Geometry check sheet. Reference: the model listing, model coordinates, mm. Face numbers are marked on the shaded views. A direction names the side the tool comes from. Round coordinates to 2 decimals unless told otherwise and drop trailing zeros. Order: outer loops, then holes, each group sorted by start corner. A loop starts at its lowest first (then second) coordinate and runs counter-clockwise, first axis right, second up.
(1) Thickness scan on L1, parallel to Z at x = 64, y = 22; L2, parallel to X at y = 3.15, z = 0; L3, parallel to Z at x = -75, y = 1.8. Record the ranges inside material, lowest first.
(2) Draft check along Z on the marked faces 1, 2 and 3. Enter one of: pulls with the +Z half, pulls with the -Z half, needs draft (parallel to the pull), parting line crosses it, or undercut.
(3) Cross-section at B-B on y = 19.25. Enter the section's corners in (x, z).
(4) Cross-section at A-A on z = 0. Enter the section's corners in (x, y).
(5) Set-up check for the marked faces 4 and 5: record each of +Z, -Z, +X, -X, +Y, -Y from which the full face is reachable in a straight line by a thin tool's end or side.
(6) Gauge pin test, flat ends, axial feed: P1, Ø5, axis at x = 62.5, z = 68.5, coming from the +Y side; P2, Ø7.5, axis at y = 20.5, z = 50.5, coming from the -X side; P3, Ø3, axis at y = 3, z = 17.5, coming from the -X side; P4, Ø2, axis at x = -8.5, z = -74.5, coming from the -Y side. Record the tip position at first contact, or that the pin passes through.
from build123d import *

# Parameters (mm, degrees)
BOSS_EXTRUDE2_DEPTH      = 4
CUT_EXTRUDE3_DEPTH       = 157.951186811
CUT_EXTRUDE3_DEPTH_BACK  = 157.951186811
SKETCH3_R                = 1.6
CUT_EXTRUDE6_DEPTH       = 157.951186811
CUT_EXTRUDE6_DEPTH_BACK  = 157.951186811
SKETCH6_R                = 17.5
SKETCH8_R                = 1.5
CUT_EXTRUDE7_DEPTH       = 4
CIRPATTERN1_COUNT        = 4
SKETCH10_R               = 1.55
CUT_EXTRUDE8_DEPTH       = 4
SKETCH11_W               = 146
SKETCH11_H               = 43.5
SKETCH11_W_2             = 140
SKETCH11_H_2             = 38
BOSS_EXTRUDE4_DEPTH      = 25
SKETCH12_W               = 90
SKETCH12_H               = 3
CUT_EXTRUDE9_DEPTH       = 25
FILLET1_R                = 2
SKETCH19_W               = 12
SKETCH19_H               = 6
CUT_EXTRUDE11_DEPTH      = 159.879435552
CUT_EXTRUDE12_DEPTH      = 159.879435552
CUT_EXTRUDE12_DEPTH_BACK = 159.879435552
SKETCH20_W               = 15
SKETCH20_H               = 15
FILLET2_R                = 25
FILLET3_R                = 4


with BuildPart() as part:
    # Sketch1 → Boss-Extrude2 (new body)
    with BuildSketch(Plane(origin=(0, 0, 0), x_dir=(1, 0, 0), z_dir=(0, 1, 0))):
        Polygon((0, -110.94520053), (78.450103635, -78.450103635), (110.94520053, 0), (78.450103635, 78.450103635), (0, 110.94520053), (-78.450103635, 78.450103635), (-110.94520053, 0), (-78.450103635, -78.450103635), align=None)
    extrude(amount=BOSS_EXTRUDE2_DEPTH)

    # Sketch3 → Cut-Extrude3 (cut, two sides: drawn at the far end of the back side and taken through both)
    with BuildSketch(Plane(origin=(0, 4, 0), x_dir=(1, 0, 0), z_dir=(0, 1, 0)).offset(-CUT_EXTRUDE3_DEPTH_BACK)):
        with Locations(Location((-75, -75, 0), (0, 0, 270))):
            Circle(SKETCH3_R)
        with Locations(Location((75, -75, 0), (0, 0, 270))):
            Circle(SKETCH3_R)
        with Locations(Location((75, 75, 0), (0, 0, 270))):
            Circle(SKETCH3_R)
        with Locations(Location((-75, 75, 0), (0, 0, 270))):
            Circle(SKETCH3_R)
    extrude(amount=CUT_EXTRUDE3_DEPTH + CUT_EXTRUDE3_DEPTH_BACK, mode=Mode.SUBTRACT)

    # Sketch6 → Cut-Extrude6 (cut, two sides: drawn at the far end of the back side and taken through both)
    with BuildSketch(Plane(origin=(0, 4, 0), x_dir=(1, 0, 0), z_dir=(0, 1, 0)).offset(-CUT_EXTRUDE6_DEPTH_BACK)):
        with Locations(Location((0, 0, 0), (0, 0, 270))):
            Circle(SKETCH6_R)
    extrude(amount=CUT_EXTRUDE6_DEPTH + CUT_EXTRUDE6_DEPTH_BACK, mode=Mode.SUBTRACT)

    # Sketch8 → Cut-Extrude7 (cut)
    with BuildSketch(Plane(origin=(0, 4, 0), x_dir=(1, 0, 0), z_dir=(0, 1, 0))):
        with Locations(Location((-15, -66.19520053, 0), (0, 0, 270))):
            Circle(SKETCH8_R)
        with Locations(Location((15, -66.19520053, 0), (0, 0, 270))):
            Circle(SKETCH8_R)
        with Locations(Location((-15, -95.94520053, 0), (0, 0, 270))):
            Circle(SKETCH8_R)
        with Locations(Location((15, -95.94520053, 0), (0, 0, 270))):
            Circle(SKETCH8_R)
    cut_extrude7 = extrude(amount=-CUT_EXTRUDE7_DEPTH, mode=Mode.SUBTRACT)

    # CirPattern1: Cut-Extrude7 ×4 about axis
    cirpattern1_axis = Axis((0, 0, 0), (0, 1, 0))
    for i in range(1, CIRPATTERN1_COUNT):
        add(cut_extrude7.rotate(cirpattern1_axis, i * 360 / CIRPATTERN1_COUNT), mode=Mode.SUBTRACT)

    # Sketch10 → Cut-Extrude8 (cut)
    with BuildSketch(Plane(origin=(0, 4, 0), x_dir=(1, 0, 0), z_dir=(0, 1, 0))):
        with Locations(Location((-50, 29, 0), (0, 0, 270))):
            Circle(SKETCH10_R)
        with Locations(Location((-50, -13, 0), (0, 0, 270))):
            Circle(SKETCH10_R)
        with Locations(Location((50, -13, 0), (0, 0, 270))):
            Circle(SKETCH10_R)
        with Locations(Location((50, 29, 0), (0, 0, 270))):
            Circle(SKETCH10_R)
        with Locations(Location((60.1, 51, 0), (0, 0, 270))):
            Circle(SKETCH10_R)
        with Locations(Location((-60.1, 61.564, 0), (0, 0, 270))):
            Circle(SKETCH10_R)
        with Locations(Location((60.1, 61.564, 0), (0, 0, 270))):
            Circle(SKETCH10_R)
        with Locations(Location((-60.1, 51, 0), (0, 0, 270))):
            Circle(SKETCH10_R)
    extrude(amount=-CUT_EXTRUDE8_DEPTH, mode=Mode.SUBTRACT)

    # Sketch11 → Boss-Extrude4 (add)
    with BuildSketch(Plane(origin=(0, 4, 0), x_dir=(1, 0, 0), z_dir=(0, 1, 0))):
        with Locations((0, -41.25)):
            Rectangle(SKETCH11_W, SKETCH11_H)
        with Locations((0, -41)):
            Rectangle(SKETCH11_W_2, SKETCH11_H_2, mode=Mode.SUBTRACT)
    extrude(amount=BOSS_EXTRUDE4_DEPTH)

    # Sketch12 → Cut-Extrude9 (cut)
    with BuildSketch(Plane(origin=(0, 29, 0), x_dir=(1, 0, 0), z_dir=(0, 1, 0))):
        Polygon((-73, -19.5), (-43, -19.5), (-43, -22), (-70, -22), (-70, -59.5), (-73, -59.5), align=None)
        with Locations((0, -61.5)):
            Rectangle(SKETCH12_W, SKETCH12_H)
    extrude(amount=-CUT_EXTRUDE9_DEPTH, mode=Mode.SUBTRACT)

    # Fillet1
    fillet1_edges = [part.edges().sort_by_distance(p)[0] for p in [
        (59, 4, 63),
        (-73, 4, 61.25),
        (73, 4, 41.25),
        (15, 4, 19.5),
        (-59, 4, 63),
    ]]
    fillet(fillet1_edges, radius=FILLET1_R - 0.0001)  # a hair under: the kernel refuses the full size

    # Sketch19 → Cut-Extrude11 (cut, through all)
    with BuildSketch(Plane(origin=(0, 4, 0), x_dir=(1, 0, 0), z_dir=(0, 1, 0))):
        with Locations((-52.000462783, -19)):
            Rectangle(SKETCH19_W, SKETCH19_H)
    extrude(amount=-CUT_EXTRUDE11_DEPTH, mode=Mode.SUBTRACT)

    # Sketch20 → Cut-Extrude12 (cut, two sides: drawn at the far end of the back side and taken through both)
    with BuildSketch(Plane(origin=(0, 4, 0), x_dir=(1, 0, 0), z_dir=(0, 1, 0)).offset(-CUT_EXTRUDE12_DEPTH_BACK)):
        with Locations((33.5, 73.69520053)):
            Rectangle(SKETCH20_W, SKETCH20_H)
    extrude(amount=CUT_EXTRUDE12_DEPTH + CUT_EXTRUDE12_DEPTH_BACK, mode=Mode.SUBTRACT)

    # Fillet2
    fillet2_edges = [part.edges().sort_by_distance(p)[0] for p in [
        (-110.94520053, 2, 0),
        (0, 2, -110.94520053),
        (110.94520053, 2, 0),
        (0, 2, 110.94520053),
    ]]
    fillet(fillet2_edges, radius=FILLET2_R)

    # Fillet3
    fillet3_edges = [part.edges().sort_by_distance(p)[0] for p in [
        (41, 2, -81.19520053),
    ]]
    fillet(fillet3_edges, radius=FILLET3_R)


solid = part.part
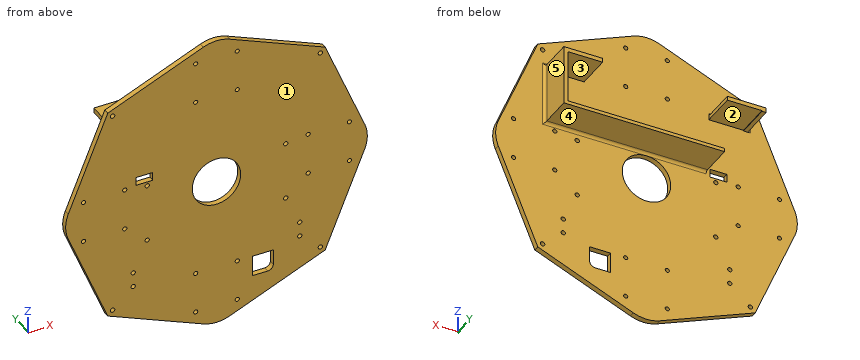
Found:
1. L1: z = 19.5 to 22, 60 to 63
1. L2: x = -108.89 to -17.5, 17.5 to 108.89
1. L3: z = -79.88 to -76.6, -73.4 to 73.4, 76.6 to 79.88
2. face 1: needs draft
2. face 2: pulls with the -Z half
2. face 3: undercut
3. outline: (-73, 59.5) - (-70, 59.5) - (-70, 60) - (-45, 60) - (-45, 63) - (-73, 63) - close; (-43, 19.5) - (73, 19.5) - (73, 63) - (45, 63) - (45, 60) - (70, 60) - (70, 22) - (-43, 22) - close
4. outline: (-108.89, 0) - (-17.5, 0) - (-17.5, 4) - (-108.89, 4) - close; (17.5, 0) - (108.89, 0) - (108.89, 4) - (17.5, 4) - close
5. face 4: -Z, +X, -X, +Y
5. face 5: +Z, -Z, +X, +Y
6. P1: stops at y = 4
6. P2: stops at x = 70
6. P3: stops at x = -104.32
6. P4: stops at y = 0
